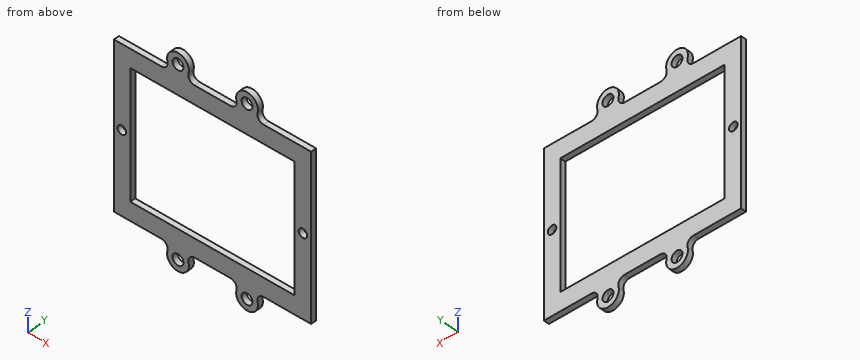
Autodesk Inventor part; units mm, degrees
ref_plane "Work Plane4" through (0, 32, 0) normal (0, 1, 0) x (-1, 0, 0)
ref_plane "YZ Plane" through (0, 0, 0) normal (1, 0, 0) x (0, 1, 0)
ref_plane "XY Plane" through (0, 0, 0) normal (0, 0, 1) x (1, 0, 0)
ref_plane "Work Plane4" through (0, 32, 0) normal (0, 1, 0) x (-1, 0, 0)
sketch "Sketch1" plane through (0, 0, 0) normal (0, 1, 0) x (-1, 0, 0)
  line L0 (33.75, 44.75) -> (-33.75, 44.75)
  line L1 (-33.75, 44.75) -> (-33.75, -44.75)
  line L2 (-33.75, -44.75) -> (33.75, -44.75)
  line L3 (33.75, -44.75) -> (33.75, 44.75)
  line L4 (21.75, -36.75) -> (-21.75, -36.75)
  line L5 (21.75, 36.75) -> (-21.75, 36.75)
  line L6 (21.75, 36.75) -> (21.75, -36.75)
  line L7 (-21.75, 36.75) -> (-21.75, -36.75)
  line L8 (33.75, -41.75) -> (-33.75, -41.75)
  line L9 (33.75, 41.75) -> (-33.75, 41.75)
  line L10 (-6.7955, 36.75) -> (21.75, 0)
  line L11 (21.75, 0) -> (0, -36.75)
  point P0 (0, 0)
  point P1 (-33.75, 0)
  dimension "d0" = 83.5
  dimension "d1" = 3
  dimension "d2" = 3
  dimension "d4" = 5
  dimension "d5" = 5
  dimension "d6" = 12
  dimension "d7" = 12
  dimension "d8" = 67.5
  dimension "d9" = 33.75
  dimension "d10" = 41.75
sketch "Sketch2" plane through (0, 32, 0) normal (0, 1, 0) x (1, 0, 0)
  line L0 (-65.75, 34.75) -> (24.75, 34.75)
  line L1 (-65.75, -34.75) -> (24.75, -34.75)
  line L2 (24.75, -34.75) -> (24.75, 34.75)
  line L3 (-65.75, -34.75) -> (-65.75, 34.75)
  line L4 (-74.75, -44.75) -> (-74.75, 44.75)
  line L5 (33.75, -44.75) -> (33.75, 44.75)
  line L6 (33.75, 44.75) -> (-33.75, 44.75)
  line L7 (-74.75, -44.75) -> (33.75, -44.75)
  line L8 (-74.75, 44.75) -> (33.75, 44.75)
  dimension "d94" = 69.5
  dimension "d96" = 90.5
  dimension "d97" = 9
  dimension "d98" = 9
  dimension "d99" = 10
  dimension "d100" = 10
extrude "Extrusion3" add sketch "Sketch2" along normal blind 3
sketch "Sketch3" plane through (0, 32, 0) normal (0, 1, 0) x (1, 0, 0)
  circle A0 centre (29.25, 0) radius 4.5
  circle A1 centre (-70.45, 0) radius 4.5
  circle A2 centre (-70.45, 0) radius 2.35
  circle A3 centre (29.25, 0) radius 2.35
  line L0 (33.75, -44.75) -> (33.75, 44.75)
  point P0 (0, 0)
  dimension "d24" = 9
  dimension "d27" = 4.7
  dimension "d43" = 99.7
  dimension "d44" = 4.5
extrude "Extrusion5" cut sketch "Sketch3" along normal blind 3 contours A2 | A3
sketch "Sketch9" plane through (0, 35, 0) normal (0, 1, 0) x (1, 0, 0)
  circle A0 centre (-39.5, -50.75) radius 3
  circle A1 centre (-39.5, -50.75) radius 6
  line L0 (-74.75, -44.75) -> (33.75, -44.75)
  circle A2 centre (-1.5, -50.75) radius 3
  circle A3 centre (-1.5, -50.75) radius 6
  arc A4 (7.6652, -44.75) -> (4.2885, -49.1711) centre (7.6652, -48.25) ccw
  arc A5 (-7.2885, -49.1711) -> (-10.6652, -44.75) centre (-10.6652, -48.25) ccw
  arc A6 (-30.3348, -44.75) -> (-33.7115, -49.1711) centre (-30.3348, -48.25) ccw
  arc A7 (-45.2885, -49.1711) -> (-48.6652, -44.75) centre (-48.6652, -48.25) ccw
  line L1 (33.75, -44.75) -> (33.75, 44.75)
  line L2 (-74.75, 44.75) -> (-74.75, -44.75)
  line L3 (64.0405, 0) -> (-151.031, 0) construction
  circle A8 centre (-39.5, 50.75) radius 3
  circle A9 centre (-39.5, 50.75) radius 6
  circle A10 centre (-1.5, 50.75) radius 3
  circle A11 centre (-1.5, 50.75) radius 6
  arc A12 (4.2885, 49.1711) -> (7.6652, 44.75) centre (7.6652, 48.25) ccw
  arc A13 (-10.6652, 44.75) -> (-7.2885, 49.1711) centre (-10.6652, 48.25) ccw
  arc A14 (-33.7115, 49.1711) -> (-30.3348, 44.75) centre (-30.3348, 48.25) ccw
  arc A15 (-48.6652, 44.75) -> (-45.2885, 49.1711) centre (-48.6652, 48.25) ccw
  line L4 (33.75, 44.75) -> (-74.75, 44.75)
  point P0 (0, 0)
  dimension "d101" = 6
  dimension "d102" = 12
  dimension "d103" = 38
  dimension "d104" = 7
  dimension "d105" = 108.5
  dimension "d106" = 35.25
extrude "Extrusion10" add sketch "Sketch9" against normal blind 3 contours A1 | A1 L0 A6 | A7 L0 A1 | L0 A3 A5 | L0 A4 A3 | A3 | A15 A9 L4 | A9 | A9 A14 L4 | L4 A11 A12 | A13 A11 L4 | A11
equation "\"d44\" = 0.5 * d24"
equation "\"d2\" = d1"
equation "\"d5\" = d4"
equation "\"d7\" = d6"
properties part number "CO-1-02-fuseMount"
Source: CAD feature listing. Evaluate the final solid. Frame: model axes, mm. Round coordinates to 2 decimals unless told otherwise and drop trailing zeros. Loops run counter-clockwise (first coordinate to the right, second up) from the corner with the lowest first, then second, coordinate; pieces in that order, holes last. Notation, with made-up numbers: (48, -37) - (93, -37) arc R33 ccw to (93, -9) - close; hole circle Ø3 at (31.25, 83). An arc over 180 degrees is marked (long way). Write item = value, one per line. Start each with the question number.
(1) Section query A-A, the plane x = -39.5. Output: boundary loops of the cut face in (y, z), plus the area to 3 significant figures.
(2) Section query D-D, the plane z = 25.5. Output: boundary loops of the cut face in (x, y), plus the area to 3 significant figures.
(3) Section query B-B, the plane z = -50.75. Output: boundary loops of the cut face in (x, y), plus the area to 3 significant figures.
(4) Pin query (flat end, axial travel): pin 1 (3.5 mm diameter, centred on x = -39.5, z = 50.75, fed in from -Y); pin 2 (1.5 mm diameter, centred on x = -32.5, y = 33, fed in from +Z); pin 3 (0.9 mm diameter, centred on x = -59, y = 34, fed in from +Z). Return the tip coordinate at first contact, or that it passes through.
(5) Ray query, line 1 along X through (y, z) = (32.45, 51); line 2 along Z through (x, y) = (-1.5, 34.15); line 3 along Z through (x, y) = (24.5, 33.9). Return the intervals inside material, ascending. Write a range as from..to.
(6) Section query C-C, the plane x = 29.25. Output: boundary loops of the cut face in (y, z), plus the area to 3 significant figures.
Conclusion:
q1.outline = (32, -56.75) - (35, -56.75) - (35, -53.75) - (32, -53.75) - close; (32, -47.75) - (35, -47.75) - (35, -34.75) - (32, -34.75) - close; (32, 34.75) - (35, 34.75) - (35, 47.75) - (32, 47.75) - close; (32, 53.75) - (35, 53.75) - (35, 56.75) - (32, 56.75) - close
q1.area = 96.0 mm2
q2.outline = (-74.75, 32) - (-65.75, 32) - (-65.75, 35) - (-74.75, 35) - close; (24.75, 32) - (33.75, 32) - (33.75, 35) - (24.75, 35) - close
q2.area = 54.0 mm2
q3.outline = (-45.5, 32) - (-42.5, 32) - (-42.5, 35) - (-45.5, 35) - close; (-36.5, 32) - (-33.5, 32) - (-33.5, 35) - (-36.5, 35) - close; (-7.5, 32) - (-4.5, 32) - (-4.5, 35) - (-7.5, 35) - close; (1.5, 32) - (4.5, 32) - (4.5, 35) - (1.5, 35) - close
q3.area = 36.0 mm2
q4.pin_1 = through
q4.pin_2 = 46.31
q4.pin_3 = 44.75
q5.line_1 = -45.49..-42.49, -36.51..-33.51, -7.49..-4.49, 1.49..4.49
q5.line_2 = -56.75..-53.75, -47.75..-34.75, 34.75..47.75, 53.75..56.75
q5.line_3 = -44.75..-34.75, 34.75..44.75
q6.outline = (32, -44.75) - (35, -44.75) - (35, -2.35) - (32, -2.35) - close; (32, 2.35) - (35, 2.35) - (35, 44.75) - (32, 44.75) - close
q6.area = 254 mm2
